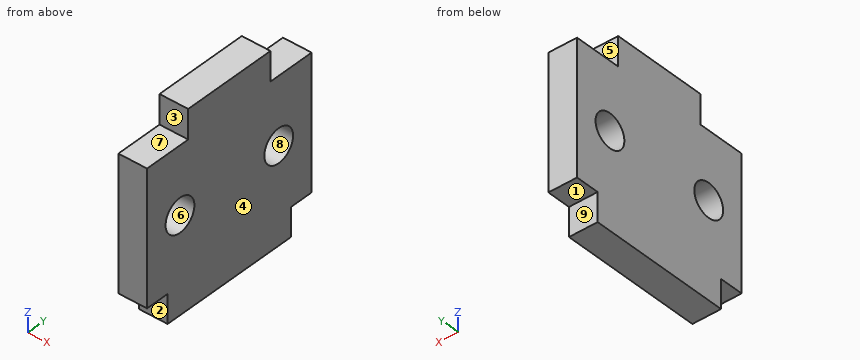
```python
from build123d import *

# Parameters (mm, degrees)
F0_W     = 15
F0_H     = 3
F0_R     = 1.75
F0_W_2   = 10
F0_H_2   = 3.05
F1_DEPTH = 3


# Not quite as in the source:
# - a feature names something its author has since deleted; it is built from what else it names


with BuildPart() as f1:
    # F0 (on Right) → F1 (new body)
    with BuildSketch(Plane.YZ):
        with Locations((0, -8.475)):
            Rectangle(F0_W, F0_H)
        Polygon((7.5, -6.975), (10, -6.975), (10, 6.975), (5, 6.975), (-5, 6.975), (-10, 6.975), (-10, -6.975), (-7.5, -6.975), align=None)
        with Locations((-6, 0)):
            Circle(F0_R, mode=Mode.SUBTRACT)
        with Locations((6, 0)):
            Circle(F0_R, mode=Mode.SUBTRACT)
        with Locations((0, 8.5)):
            Rectangle(F0_W_2, F0_H_2)
    extrude(amount=F1_DEPTH)


solid = f1.part
```
The model under review builds one solid part; all positions refer to its coordinate system, in mm. Face numbers are marked on the shaded views. A direction names the side the tool comes from. Give positions to 0.01 mm unless a question says otherwise; leave off trailing zeros. Write each loop counter-clockwise with the first axis right and the second up, starting at its lowest first coordinate (ties: lowest second). Pieces come first, ordered by that corner, then holes. Notation, with made-up numbers: M 51,-33.5 L 55,-33.5 A17 ccw 55,-7.5 Z; hole C 9.5,-40 d11. An arc over 180 degrees is marked long. Write item = value, one per line. Start each with the question number.
Q1. For line 1 (Y direction, x = 1.6, z = 9); line 2 (Z direction, x = 2, y = 6) (3 decimals); line 3 (Z direction, x = 2.3, y = -7) (3 decimals), list the stretches that pass through material, from the lowest coordinate up.
Q2. We need section C-C (x = 0.75). State the section outline as (y, z) points (3 decimals).
Q3. We need section B-B (z = 0). State the section outline as (x, y) points, plus the area to 3 significant figures.
Q4. Clearance check with flat-ended pins moving along their axes: pin 1 (1.2 mm diameter, centred on x = 2, y = 9, fed in from -Z) (3 decimals); pin 2 (1.5 mm diameter, centred on x = 2, z = 8.5, fed in from -Y); pin 3 (1.5 mm diameter, centred on x = 2, y = 8, fed in from +Z) (3 decimals); pin 4 (3 mm diameter, centred on y = 6, z = 0, fed in from -X). State where each tip first meets the part, or that it passes through.
Q5. We need section A-A (y = -6). State the section outline as (x, z) points (3 decimals), plus the area to 4 significant figures.
Q6. Machinability: for the marked faces 1, 2, 3, 4 and 5, which of the approach directions +Z, -Z, +X, -X, +Y, -Y give a long, thin tool a straight path to every point of the face, cutting with its end or side? Answer none if there is none.
Q7. Mouldability with a two-part tool opening along Y and no side actions: class the marked faces 6, 7, 8 and 9 as released by +Y, released by -Y, zero draft, split by the parting line, or undercut.
Q8. We need section D-D (z = -8.5). State the section outline as (x, y) points.
Result set:
q1.line_1 = -5 to 5
q1.line_2 = -9.975 to -1.75, 1.75 to 6.975
q1.line_3 = -9.975 to -1.436, 1.436 to 6.975
q2.outline = M -10,-6.975 L -7.5,-6.975 L -7.5,-9.975 L 7.5,-9.975 L 7.5,-6.975 L 10,-6.975 L 10,6.975 L 5,6.975 L 5,10.025 L -5,10.025 L -5,6.975 L -10,6.975 Z; hole C -6,0 d3.5; hole C 6,0 d3.5
q3.outline = M 0,-10 L 3,-10 L 3,-7.75 L 0,-7.75 Z; M 0,-4.25 L 3,-4.25 L 3,4.25 L 0,4.25 Z; M 0,7.75 L 3,7.75 L 3,10 L 0,10 Z
q3.area = 39.0 mm2
q4.pin_1 = -6.975
q4.pin_2 = -5
q4.pin_3 = 6.975
q4.pin_4 = through
q5.outline = M 0,-9.975 L 3,-9.975 L 3,-1.75 L 0,-1.75 Z; M 0,1.75 L 3,1.75 L 3,6.975 L 0,6.975 Z
q5.area = 40.35 mm2
q6.face_1 = -Z, +X, -X, +Y
q6.face_2 = -Z, +X, -X, -Y
q6.face_3 = +Z, +X, -X, -Y
q6.face_4 = +Z, -Z, +X, +Y, -Y
q6.face_5 = +Z, +X, -X, +Y
q7.face_6 = undercut
q7.face_7 = zero draft
q7.face_8 = undercut
q7.face_9 = released by +Y
q8.outline = M 0,-7.5 L 3,-7.5 L 3,7.5 L 0,7.5 Z
